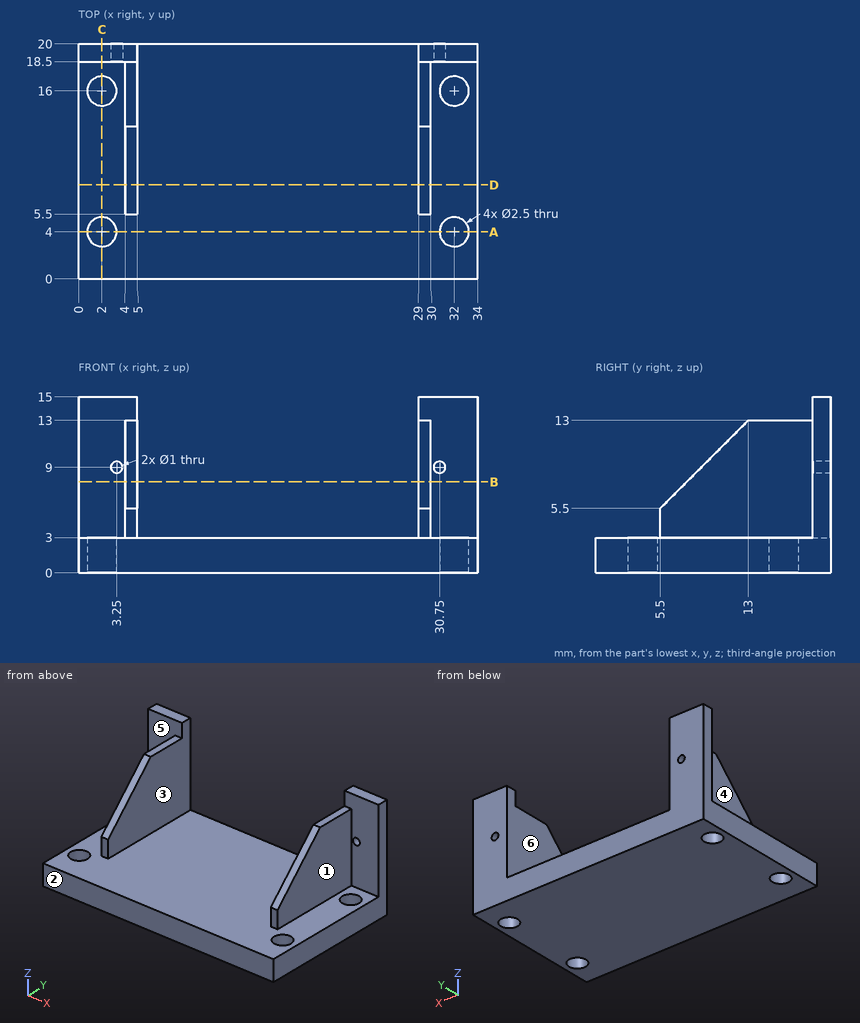
For this review, use the dimensioned drawing (mm, ordinates from the lowest corner) and the shaded views. A direction names the side the tool comes from. Round coordinates to 2 decimals unless told otherwise and drop trailing zeros. Order: outer loops, then holes, each group sorted by start corner. A loop starts at its lowest first (then second) coordinate and runs counter-clockwise, first axis right, second up. Notation, with made-up numbers: M 3.5,-35 L 50.5,-35 A3 ccw 50.5,-30 Z; hole C -7,63 d9. An arc over 180 degrees is marked long. Use a Markdown table: item, result. Add a question column.
Item 1: Add section D-D, the plane y = 8. Give the boundary of the cut face in (x, z), then the cut area to 3 significant figures.
Item 2: Add section B-B, the plane z = 7.75. Give the boundary of the cut face in (x, y).
Item 3: Tool access review of the marked faces 1, 2 and 3: name each direction out of +Z, -Z, +X, -X, +Y, -Y from which nothing blocks a thin tool from reaching the whole face with its end or side.
Item 4: Mouldability with a two-part tool opening along X and no side actions: class the marked faces 4, 5 and 6 as released by +X, released by -X, zero draft, split by the parting line, or undercut.
Item 5: Insertion check: pin 1 (2 mm diameter, centred on x = 2, y = 4, fed in from +Z); pin 2 (3 mm diameter, centred on y = 14, z = 6, fed in from -X); pin 3 (3 mm diameter, centred on x = 32, y = 16, fed in from +Z); pin 4 (1.1 mm diameter, centred on x = 4.5, z = 4.5, fed in from -Y). Each pin has a flat end and moves straight along its axis. Give the tip position at first contact, or say it passes through.
Item 6: To check wall thickness, follow line 1 along Y through (x, z) = (32, 0.9); line 2 along X through (y, z) = (14.5, 9.75); line 3 along Z through (x, y) = (3.25, 19.25). State the ranges of each line that lie inside material, in increasing order.
Item 7: Add section A-A, the plane y = 4. Give the boundary of the cut face in (x, z), then the cut area to 3 significant figures.
Item 8: Add section C-C, the plane x = 2. Give the boundary of the cut face in (y, z).
Geometry results:
| question | item | result |
|---|---|---|
| 1 | outline | M 0,0 L 34,0 L 34,3 L 30,3 L 30,8 L 29,8 L 29,3 L 5,3 L 5,8 L 4,8 L 4,3 L 0,3 Z |
| 1 | area | 112 mm² |
| 2 | outline | M 0,18.5 L 4,18.5 L 4,7.75 L 5,7.75 L 5,20 L 0,20 Z; M 29,7.75 L 30,7.75 L 30,18.5 L 34,18.5 L 34,20 L 29,20 Z |
| 3 | face 1 | +Z, +X, -Y |
| 3 | face 2 | +Z, -Z, +X, -X, -Y |
| 3 | face 3 | +Z, +Y, -Y |
| 4 | face 4 | released by -X |
| 4 | face 5 | zero draft |
| 4 | face 6 | undercut |
| 5 | pin 1 | passes through |
| 5 | pin 2 | stops at x = 4 |
| 5 | pin 3 | stops at z = 3 |
| 5 | pin 4 | stops at y = 5.5 |
| 6 | line 1 | y = 0 to 2.75, 5.25 to 14.75, 17.25 to 20 |
| 6 | line 2 | x = 4 to 5, 29 to 30 |
| 6 | line 3 | z = 0 to 8.5, 9.5 to 15 |
| 7 | outline | M 0,0 L 0.75,0 L 0.75,3 L 0,3 Z; M 3.25,0 L 30.75,0 L 30.75,3 L 3.25,3 Z; M 33.25,0 L 34,0 L 34,3 L 33.25,3 Z |
| 7 | area | 87.0 mm² |
| 8 | outline | M 0,0 L 2.75,0 L 2.75,3 L 0,3 Z; M 5.25,0 L 14.75,0 L 14.75,3 L 5.25,3 Z; M 17.25,0 L 20,0 L 20,15 L 18.5,15 L 18.5,3 L 17.25,3 Z |
